```python
from build123d import *

# Parameters (mm, degrees)
PAD_DEPTH    = 6
SKETCH_W     = 25
SKETCH_H     = 8.532326
PAD001_DEPTH = 14
SKETCH002_R  = 2
POCKET_DEPTH = 25.001


with BuildPart() as part:
    # Sketch001 → Pad (new body)
    with BuildSketch(Plane.XY):
        with BuildLine():
            Line((0, -0.513451), (12.5, -0.513451))
            Line((12.5, -0.513451), (12.5, 8.018875))
            Line((12.5, 8.018875), (5.444822, 8.018875))
            Line((5.444822, 8.018875), (2.947073, 22.018734))
            ThreePointArc((2.947073, 22.018734), (1.921936, 23.788122), (0, 24.486549))
            ThreePointArc((0, 24.486549), (-1.921936, 23.788122), (-2.947073, 22.018734))
            Line((-5.444822, 8.018875), (-2.947073, 22.018734))
            Line((-12.5, 8.018875), (-5.444822, 8.018875))
            Line((-12.5, -0.513451), (-12.5, 8.018875))
            Line((0, -0.513451), (-12.5, -0.513451))
        make_face()
    extrude(amount=PAD_DEPTH)

    # Sketch → Pad001 (new body)
    with BuildSketch(Plane.XY.offset(6)):
        with Locations((0, 3.752712)):
            Rectangle(SKETCH_W, SKETCH_H)
    extrude(amount=PAD001_DEPTH)

    # Sketch002 → Pocket (cut, through all)
    with BuildSketch(Plane.XZ.offset(0.513451)):
        with Locations((-7.711432, 15.261821)):
            Circle(SKETCH002_R)
        with Locations((7.711432, 15.261821)):
            Circle(SKETCH002_R)
    extrude(amount=-POCKET_DEPTH, mode=Mode.SUBTRACT)


solid = part.part
```
Check sheet for the modelled part. Datum: model origin and axes. Units: mm. A direction names the side the tool comes from. Give positions to 0.01 mm unless a question says otherwise; leave off trailing zeros. Loops run counter-clockwise (first coordinate to the right, second up) from the corner with the lowest first, then second, coordinate; pieces in that order, holes last. Notation, with made-up numbers: M 7,74.25 L 39,74.25 A29 ccw 39,106.25 Z; hole C 71.25,24 d5. An arc over 180 degrees is marked long. Answer as CSV lines item,"result".
Item 1: Set-up check for faces 4 (the face through (0, 9, 0)), 5 (the face through (0, 15, 6)): record each of +Z, -Z, +X, -X, +Y, -Y from which the full face is reachable in a straight line by a thin tool's end or side.
Reply:
face 4,"-Z, +X, -X, +Y, -Y"
face 5,"+Z, +X, -X, +Y"
Item 2: Sectioned sample at C-C, the plane y = 2. Enter the section's corners in (x, z), then the cut area to 3 significant figures.
Reply:
outline,"M -12.5,0 L 12.5,0 L 12.5,20 L -12.5,20 Z; hole C -7.71,15.26 d4; hole C 7.71,15.26 d4"
area,"475 mm^2"
Item 3: Sectioned sample at D-D, the plane z = 12. Enter the section's corners in (x, y).
Reply:
outline,"M -12.5,-0.51 L 12.5,-0.51 L 12.5,8.02 L -12.5,8.02 Z"
Item 4: Scan lines: L1, parallel to Y at x = -7.75, z = 9.75; L2, parallel to Z at x = -1, y = 20.25; L3, parallel to Z at x = 8.75, y = 5.5. Record each from-to range of solid material in increasing order.
Reply:
L1,"-0.51 to 8.02"
L2,"0 to 6"
L3,"0 to 13.55, 16.97 to 20"
Item 5: Depth check by flat-ended pin: pin 1 Ø8.5 at (x, y) = (0.5, 15) entering from +Z; pin 2 Ø6 at (x, z) = (4, 5) entering from +Y; pin 3 Ø3 at (y, z) = (14.5, 7) entering from +X. Enter the tip coordinate at first touch or a pass-through.
Reply:
pin 1,"z = 6"
pin 2,"y = 24.31"
pin 3,"x = 4.49"
Item 6: Draft check along Z on faces 1 (the face through (12.5, 4, 10)), 2 (the face through (-6.64, 3.69, 16.95)), 3 (the face through (0, 4, 20)). Enter one of: pulls with the +Z half, pulls with the -Z half, needs draft (parallel to the pull), parting line crosses it, or undercut.
Reply:
face 1,"needs draft"
face 2,"undercut"
face 3,"pulls with the +Z half"
Item 7: Sectioned sample at B-B, the plane x = -1. Enter the section's corners in (y, z).
Reply:
outline,"M -0.51,0 L 24.31,0 L 24.31,6 L 8.02,6 L 8.02,20 L -0.51,20 Z"
Item 8: Sectioned sample at A-A, the plane z = 16.25. Enter the section's corners in (x, y).
Reply:
outline,"M -12.5,-0.51 L -9.45,-0.51 L -9.45,8.02 L -12.5,8.02 Z; M -5.97,-0.51 L 5.97,-0.51 L 5.97,8.02 L -5.97,8.02 Z; M 9.45,-0.51 L 12.5,-0.51 L 12.5,8.02 L 9.45,8.02 Z"
